Print and shaded views of the part. All mm, measured from the part's lowest x, y and z. A direction names the side the tool comes from. Coordinates: 2 decimals unless noted, no trailing zeros. Loops run counter-clockwise (first coordinate to the right, second up) from the corner with the lowest first, then second, coordinate; pieces in that order, holes last. Notation, with made-up numbers: M 48,58.5 L 72,58.5 A26 cw 72,82.5 Z; hole C 74.5,74 d1. An arc over 180 degrees is marked long. Answer as a JSON object with one key per item and string values. Group by question number.
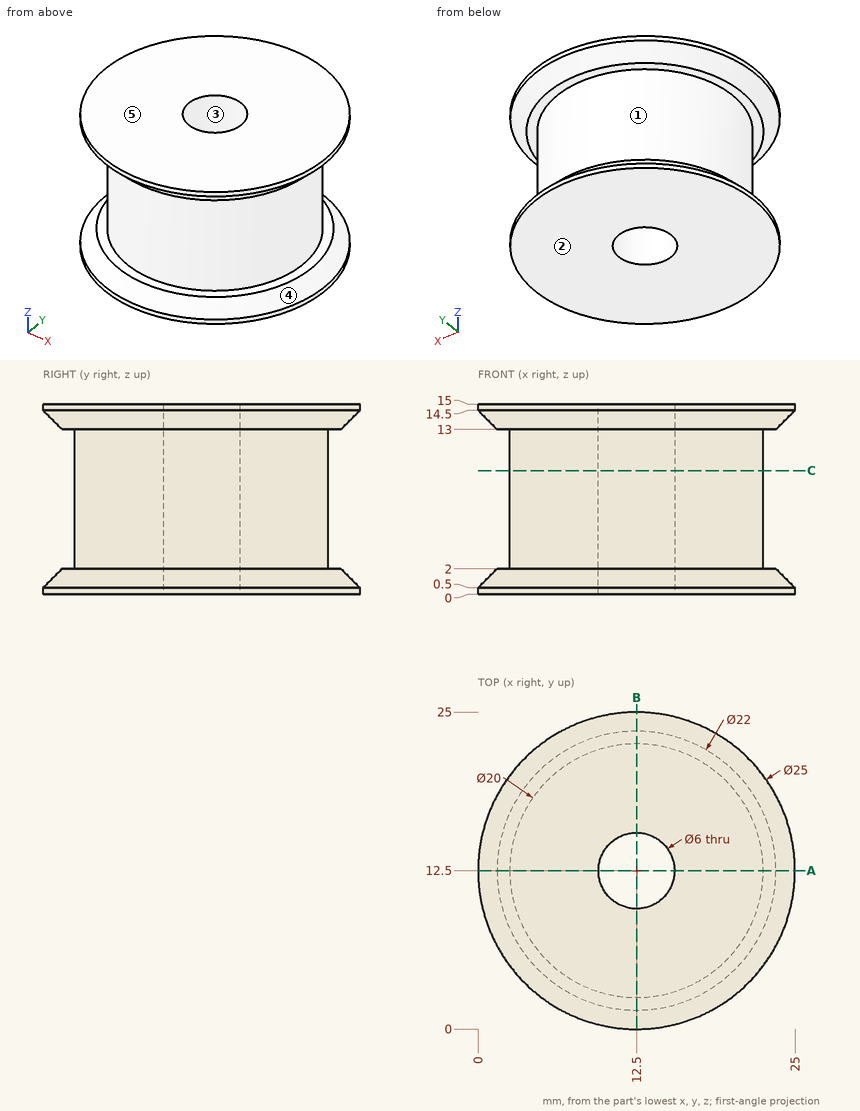
Item 1: Pull direction X, two halves, no side cores. Call the marked faces 1, 2 and 3: released by +X, released by -X, zero draft, split by the parting line, or undercut.
Item 2: Tool access for the marked faces 4 and 5: list every direction of +Z, -Z, +X, -X, +Y, -Y with a clear straight run to the whole face (end or side of a thin tool).
Item 3: Drill centre lines: L1, parallel to Z at x = 9.5, y = 23; L2, parallel to Y at x = 12.5, z = 8.75; L3, parallel to X at y = 13.5, z = 8. Where is each one in solid material? Low to high. Write a range as from..to.
Item 4: Pin check, flat tips, straight feed: pin 1 (8 mm diameter, centred on x = 9, z = 12, fed in from +Y); pin 2 (1 mm diameter, centred on x = 18.5, z = 6, fed in from +Y); pin 3 (1 mm diameter, centred on y = 15, z = 10, fed in from -X). Stop position of each tip, or through.
Item 5: Slice it at A-A, the plane y = 12.5. Write the cut outline in (x, z), then the cut area to 4 significant figures.
Item 6: Slice it at C-C, the plane z = 9.75. Write the cut outline in (x, y).
Computed:
{
 "1": {"face 1": "split by the parting line", "face 2": "zero draft", "face 3": "undercut"},
 "2": {"face 4": "none", "face 5": "+Z, +X, -X, +Y, -Y"},
 "3": {"L1": "0..2, 13..15", "L2": "2.5..9.5, 15.5..22.5", "L3": "2.55..9.67, 15.33..22.45"},
 "4": {"pin 1": "y = 24.99", "pin 2": "y = 20.85", "pin 3": "x = 2.7"},
 "5": {"outline": "M 0,0 L 9.5,0 L 9.5,15 L 0,15 L 0,14.5 L 1.5,13 L 2.5,13 L 2.5,2 L 1.5,2 L 0,0.5 Z; M 15.5,0 L 25,0 L 25,0.5 L 23.5,2 L 22.5,2 L 22.5,13 L 23.5,13 L 25,14.5 L 25,15 L 15.5,15 Z", "area": "225.5 mm2"},
 "6": {"outline": "C 12.5,12.5 d20; hole C 12.5,12.5 d6"}
}
